CAD build for the part. Positions are in the model's coordinates, mm. Face numbers are marked on the shaded views. Coordinates: 2 decimals unless noted, no trailing zeros. Write each loop counter-clockwise with the first axis right and the second up, starting at its lowest first coordinate (ties: lowest second). Pieces come first, ordered by that corner, then holes. Notation, with made-up numbers: (-22.5, 89) - (-8.5, 89) arc R20 cw to (-8.5, 126) - close; hole circle Ø2 at (-23, 23). An arc over 180 degrees is marked (long way). Answer in a Markdown table with one row per item. Add a question column.
Q1. Band-saw the part on A-A (x = 0). List the corners of the cut face in (y, z), and give its area (3 significant figures).
Q2. Two-plate mould, pull along Z, no slides. Class the marked faces 1, 2 and 3: +Z half, -Z half, draft (parallel to the pull), parting line (faces both ways), or undercut.
Q3. Pin check, flat tips, straight feed: pin 1 (1 mm diameter, centred on x = 1.5, z = 3.5, fed in from -Y); pin 2 (14.5 mm diameter, centred on x = 2.5, z = 0.5, fed in from +Y); pin 3 (11.5 mm diameter, centred on x = 0, z = 0, fed in from -Y). Stop position of each tip, or through.
Q4. Drill centre lines: line 1 along X through (y, z) = (1.9, -3); line 2 along X through (y, z) = (1.95, 4.5); line 3 along Z through (x, y) = (-3.5, 3.25). Where is each one in solid material? Low to high. Write a range as from..to.
Q5. Band-saw the part on C-C (y = 1.55). List the corners of the cut face in (x, z).
Q6. Band-saw the part on B-B (z = 0). List the corners of the cut face in (x, y), and give its area (3 significant figures).
```python
from build123d import *


with BuildPart() as part:
    # Sketch1 → Revolve1 (revolve)
    with BuildSketch(Plane.XY, mode=Mode.PRIVATE) as revolve1_sk:
        with BuildLine():
            Line((5, 1.176406116), (9.93722571, 1.176406116))
            ThreePointArc((9.93722571, 1.176406116), (10.997892387, 1.480827689), (11.735669245, 2.301419916))
            Line((11.735669245, 2.301419916), (12.23830631, 3.334538358))
            ThreePointArc((12.23830631, 3.334538358), (12.242904148, 3.410936815), (12.192133443, 3.468209845))
            Line((12.192133443, 3.468209845), (11.023145145, 4.036950875))
            ThreePointArc((11.023145145, 4.036950875), (10.946746688, 4.041548713), (10.889473658, 3.990778008))
            Line((10.889473658, 3.990778008), (10.797346375, 3.801419916))
            ThreePointArc((10.797346375, 3.801419916), (10.059569517, 2.980827689), (8.99890284, 2.676406116))
            Line((8.99890284, 2.676406116), (5, 2.676406116))
            Line((5, 2.676406116), (5, 1.176406116))
        make_face()
    revolve(revolve1_sk.sketch.rotate(Axis((0, 4.371150449, 0), (0, -1, 0)), 90), axis=Axis((0, 4.371150449, 0), (0, -1, 0)))


solid = part.part
```
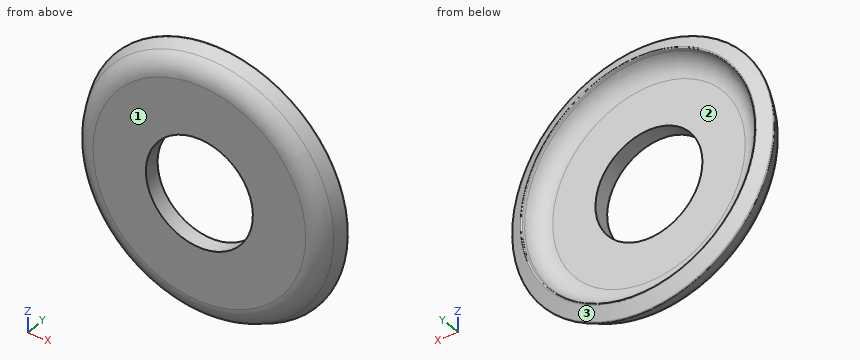
Checked values:
| question | item | result |
|---|---|---|
| 1 | outline | (1.18, -9.94) arc R2 ccw to (2.3, -11.74) - (3.33, -12.24) arc R0.1 ccw to (3.47, -12.19) - (4.04, -11.02) arc R0.1 ccw to (3.99, -10.89) - (3.8, -10.8) arc R2 cw to (2.68, -9) - (2.68, -5) - (1.18, -5) - close; (1.18, 5) - (2.68, 5) - (2.68, 9) arc R2 cw to (3.8, 10.8) - (3.99, 10.89) arc R0.1 ccw to (4.04, 11.02) - (3.47, 12.19) arc R0.1 ccw to (3.33, 12.24) - (2.3, 11.74) arc R2 ccw to (1.18, 9.94) - close |
| 1 | area | 23.2 mm² |
| 2 | face 1 | draft |
| 2 | face 2 | undercut |
| 2 | face 3 | parting line |
| 3 | pin 1 | passes through |
| 3 | pin 2 | stops at y = 2.84 |
| 3 | pin 3 | stops at y = 1.18 |
| 4 | line 1 | x = -11.08..-4, 4..11.08 |
| 4 | line 2 | x = -10.6..-2.18, 2.18..10.6 |
| 4 | line 3 | z = -11.68..-9.79, 9.79..11.68 |
| 5 | outline | circle Ø22.2 at (0, 0); hole circle Ø10 at (0, 0) |
| 6 | outline | (-12.24, 3.33) - (-11.74, 2.3) arc R2 ccw to (-9.94, 1.18) - (-5, 1.18) - (-5, 2.68) - (-9, 2.68) arc R2 cw to (-10.8, 3.8) - (-10.89, 3.99) arc R0.1 ccw to (-11.02, 4.04) - (-12.19, 3.47) arc R0.1 ccw to start; (5, 1.18) - (9.94, 1.18) arc R2 ccw to (11.74, 2.3) - (12.24, 3.33) arc R0.1 ccw to (12.19, 3.47) - (11.02, 4.04) arc R0.1 ccw to (10.89, 3.99) - (10.8, 3.8) arc R2 cw to (9, 2.68) - (5, 2.68) - close |
| 6 | area | 23.2 mm² |
